Here's how the part is built. I have some questions about the finished solid (model axes, mm). Face numbers are marked on the shaded views. Round coordinates to 2 decimals unless told otherwise and drop trailing zeros. Order: outer loops, then holes, each group sorted by start corner. A loop starts at its lowest first (then second) coordinate and runs counter-clockwise, first axis right, second up. Notation, with made-up numbers: (25, 29) -> (73, 29) arc R19 cw to (73, 61) -> close; hole circle Ø5 at (-1, 33). An arc over 180 degrees is marked (long way). One line per item, written item: value.
```python
from build123d import *

# Parameters (mm, degrees)
SKETCH2_W           = 78
SKETCH2_H           = 73
BOSS_EXTRUDE1_DEPTH = 4
SKETCH3_W           = 72
SKETCH3_H           = 67
CUT_EXTRUDE1_DEPTH  = 2
FILLET1_R           = 2


with BuildPart() as part:
    # Sketch2 → Boss-Extrude1 (new body)
    with BuildSketch(Plane(origin=(0, 0, 0), x_dir=(1, 0, 0), z_dir=(0, 1, 0))):
        with Locations((39, 36.5)):
            Rectangle(SKETCH2_W, SKETCH2_H)
    extrude(amount=BOSS_EXTRUDE1_DEPTH)

    # Sketch3 → Cut-Extrude1 (cut)
    with BuildSketch(Plane(origin=(0, 4, 0), x_dir=(1, 0, 0), z_dir=(0, 1, 0))):
        with Locations((39, 36.5)):
            Rectangle(SKETCH3_W, SKETCH3_H)
    extrude(amount=-CUT_EXTRUDE1_DEPTH, mode=Mode.SUBTRACT)

    # Fillet1
    fillet1_edges = [part.edges().sort_by_distance(p)[0] for p in [
        (39, 0, -73),
        (78, 0, -36.5),
        (39, 0, 0),
        (0, 0, -36.5),
    ]]
    fillet(fillet1_edges, radius=FILLET1_R)


solid = part.part
```
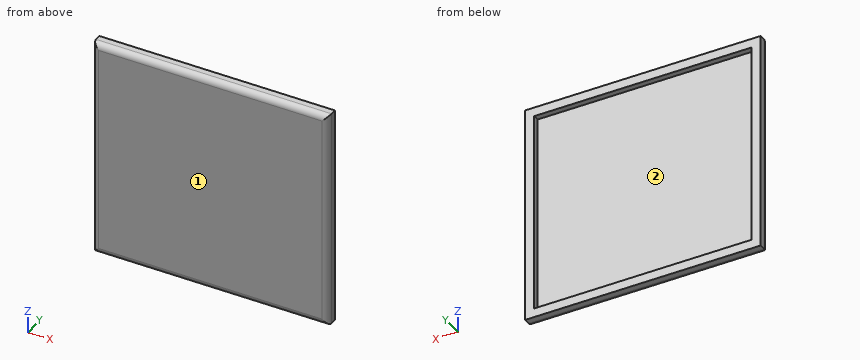
Q1. I want a section at A-A on y = 2.9. Write out the boundary of the cut face in (x, z).
Answers:
outline: (0, -73) -> (78, -73) -> (78, 0) -> (0, 0) -> close; hole (3, -70) -> (75, -70) -> (75, -3) -> (3, -3) -> close
Q2. If we mould it in two halves opening along X, with no side actions, what happens to the marked faces 1 and 2? For each: pulls with the +X half, pulls with the -X half, needs draft (parallel to the pull), parting line crosses it, or undercut.
Answers:
face 1: needs draft
face 2: undercut
Q3. For P1, Ø1.5, axis at y = 0.5, z = -16, coming from the -X side; P2, Ø1.5, axis at x = 13, z = -22.5, coming from the +Y side, each with a flat end and sliding along its axis, tell me the tip position at first contact or that it passes through.
Answers:
P1: x = 0.15
P2: y = 2
Q4. I want a section at C-C on z = -45. Write out the boundary of the cut face in (x, y).
Answers:
outline: (0, 2) arc R2 ccw to (2, 0) -> (76, 0) arc R2 ccw to (78, 2) -> (78, 4) -> (75, 4) -> (75, 2) -> (3, 2) -> (3, 4) -> (0, 4) -> close
Q5. I need wall thicknesses on line 1 along X through (y, z) = (2.2, -61); line 2 along Z through (x, y) = (54.5, 3.05); line 3 along Y through (x, z) = (47, -49.5). Which ranges of each line are inside material? Lowest first, please.
Answers:
line 1: 0 to 3, 75 to 78
line 2: -73 to -70, -3 to 0
line 3: 0 to 2
Q6. I want a section at B-B on x = 53.5. Write out the boundary of the cut face in (y, z).
Answers:
outline: (0, -71) arc R2 ccw to (2, -73) -> (4, -73) -> (4, -70) -> (2, -70) -> (2, -3) -> (4, -3) -> (4, 0) -> (2, 0) arc R2 ccw to (0, -2) -> close
